Source: CAD feature listing. Evaluate the final solid. Frame: model axes, mm. Coordinates: 2 decimals unless noted, no trailing zeros. Order: outer loops, then holes, each group sorted by start corner. A loop starts at its lowest first (then second) coordinate and runs counter-clockwise, first axis right, second up. Notation, with made-up numbers: (64, 6) - (83, 6) arc R8 cw to (83, 11) - close; hole circle Ø2 at (-16.5, 65). An arc over 180 degrees is marked (long way). One line per question, with ' | ' between items. Start each with the question number.
(1) Section B-B (z = 11). Return the cut outline in (x, y) (3 decimals).
(2) Line query: line 1 along Y through (x, z) = (0, 5.25); line 2 along X through (y, z) = (-6, 3.25); line 3 along Y through (x, z) = (8, 1.75). Output: solid intervals per line, ascending.
(3) Section C-C (x = 6). Return the cut outline in (y, z), then the cut area to 3 significant figures.
(4) Contact query for flat-ended pins moving along their axis: P1, Ø4, axis at x = 14.5, z = 8, coming from the +Y side; P2, Ø5, axis at y = 7.5, z = 7.5, coming from the -X side; P3, Ø1.5, axis at y = -4, z = 11.5, coming from the +X side. Output: stop coordinate, or through.
(5) Draft query along X for faces 1 (the flat face through (13.9, 7.88, 6.92)), 2 (the cylindrical face through (0.13, -15.69, 13.7)), 3 (the cylindrical face through (2.38, -10.74, 6.9)), 4 (the flat face through (-13.9, -7.88, 6.92)). Return one class per face: +X half, -X half, draft (parallel to the pull), parting line (faces both ways), or undercut.
(6) Section A-A (x = 0). Return the cut outline in (y, z).
from build123d import *

# Parameters (mm, degrees)
EXTRUDE_1_DEPTH     = 14
SKETCH_3_R          = 11
CUT_EXTRUDE_2_DEPTH = 29.13724178
FILLET_1_R          = 1


with BuildPart() as part:
    # 草图2 → 拉伸1 (new body)
    with BuildSketch(Plane.XY):
        Polygon((9.225, -15.9781687), (18.45, 0), (9.225, 15.9781687), (-9.225, 15.9781687), (-18.45, 0), (-9.225, -15.9781687), align=None)
    extrude(amount=EXTRUDE_1_DEPTH)

    # 草图3 → 拉伸2 (cut, through all)
    with BuildSketch(Plane(origin=(0, 0, 0), x_dir=(-1, 0, 0), z_dir=(0, 0, -1))):
        Circle(SKETCH_3_R)
    extrude(amount=-CUT_EXTRUDE_2_DEPTH, mode=Mode.SUBTRACT)

    # 圆角1
    fillet_1_edges = [part.edges().sort_by_distance(p)[0] for p in [
        (13.8375, 7.98908435, 14),
        (0, 15.9781687, 14),
        (-13.8375, 7.98908435, 14),
        (-13.8375, -7.98908435, 14),
        (0, -15.9781687, 14),
        (-13.8375, -7.98908435, 0),
        (-13.8375, 7.98908435, 0),
        (0, 15.9781687, 0),
        (13.8375, -7.98908435, 14),
        (13.8375, 7.98908435, 0),
        (13.8375, -7.98908435, 0),
        (0, -15.9781687, 0),
    ]]
    fillet(fillet_1_edges, radius=FILLET_1_R)


solid = part.part
Response values:
1) outline: (-18.45, 0) - (-9.225, -15.978) - (9.225, -15.978) - (18.45, 0) - (9.225, 15.978) - (-9.225, 15.978) - close; hole circle Ø22 at (0, 0)
2) line 1: y = -15.98 to -11, 11 to 15.98 | line 2: x = -14.99 to -9.22, 9.22 to 14.99 | line 3: y = -15.98 to -7.55, 7.55 to 15.98
3) outline: (-15.98, 1) arc R1 ccw to (-14.98, 0) - (-9.22, 0) - (-9.22, 14) - (-14.98, 14) arc R1 ccw to (-15.98, 13) - close; (9.22, 0) - (14.98, 0) arc R1 ccw to (15.98, 1) - (15.98, 13) arc R1 ccw to (14.98, 14) - (9.22, 14) - close | area: 188 mm²
4) P1: stops at y = 10.31 | P2: stops at x = -15.56 | P3: stops at x = 16.57
5) face 1: +X half | face 2: draft | face 3: undercut | face 4: -X half
6) outline: (-15.98, 1) arc R1 ccw to (-14.98, 0) - (-11, 0) - (-11, 14) - (-14.98, 14) arc R1 ccw to (-15.98, 13) - close; (11, 0) - (14.98, 0) arc R1 ccw to (15.98, 1) - (15.98, 13) arc R1 ccw to (14.98, 14) - (11, 14) - close
